Check sheet for the modelled part. Datum: model origin and axes. Units: mm. A direction names the side the tool comes from. Coordinates: 2 decimals unless noted, no trailing zeros. Loops run counter-clockwise (first coordinate to the right, second up) from the corner with the lowest first, then second, coordinate; pieces in that order, holes last. Notation, with made-up numbers: (81.25, 13) - (104.25, 13) arc R24 cw to (104.25, 43) - close; hole circle Ø8 at (-1.75, 1.5). An arc over 180 degrees is marked (long way). Use a Markdown table: item, result. Add a question column.
1) Sectioned sample at C-C, the plane y = 0.65. State how many separate pieces and enclosed holes the cut face has, then the cut area to 3 significant figures.
2) Tool access check on faces 5 (the cylindrical face through (171.507, 1.014, -95.283)), 6 (the flat face through (110, 0, -21)). Record the directions out of +Z, -Z, +X, -X, +Y, -Y that give a thin tool (end or side, any length) a straight path to the whole face; none if there is none.
3) Sectioned sample at A-A, the plane x = 58. Enter the section's corners in (y, z), then the cut area to 3 significant figures.
4) Draft check along X on faces 1 (the cylindrical face through (37.467, 1.014, -69.208)), 2 (the flat face through (201.842, 0.986, 25.333)), 3 (the cylindrical face through (173.347, 1.014, -44.294)), 4 (the flat face through (15.98, 0.99, 25.77)). Enter one of: pulls with the +X half, pulls with the -X half, needs draft (parallel to the pull), parting line crosses it, or undercut.
5) Thickness scan on line 1 (Z direction, x = 96.5, y = 0.3); line 2 (Z direction, x = 72, y = 0.1); line 3 (X direction, y = 1.15, z = -95.5). Record the ranges inside material, lowest first.
6) Go/stop test with flat-tipped pins: P1, Ø2, axis at x = 7.5, z = -9.02, coming from the +Y side; P2, Ø0.6, axis at x = 3.5, y = 1, coming from the -Z side; P3, Ø0.6, axis at y = 1, z = 37, coming from the -X side; P4, Ø1, axis at y = 1, z = -74, coming from the -X side. Record where each tip stops, or that it passes through.
7) Sectioned sample at B-B, the plane x = 17. Enter the section's corners in (y, z), then the cut area to 3 significant figures.
from build123d import *

# Parameters (mm, degrees)
SKETCH_1_R          = 1.7
EXTRUDE_1_DEPTH     = 2
SKETCH_3_R          = 3
CUT_EXTRUDE_1_DEPTH = 10
CUT_EXTRUDE_2_DEPTH = 10


with BuildPart() as part:
    # 草图1 → 凸台-拉伸1 (new body)
    with BuildSketch(Plane(origin=(0, 0, 0), x_dir=(1, 0, 0), z_dir=(0, 1, 0))):
        Polygon((0, -9.790421162), (0, 32.375054838), (13, 32.375054838), (13, 102.375054838), (0, 102.375054838), (0, 144.54053128), (31.526911935, 176.067443214), (73.692388376, 176.067443215), (73.692388376, 163.067443215), (143.692388376, 163.067443215), (143.692388376, 176.067443215), (185.857864376, 176.067443214), (217.384776311, 144.54053128), (217.384776311, 102.375054838), (204.384776311, 102.375054838), (204.384776311, 32.375054838), (217.384776311, 32.375054838), (217.384776311, -9.790421162), (185.857864376, -41.317333096), (143.692388376, -41.317333096), (143.692388376, -26.317333096), (73.692388376, -26.317333096), (73.692388376, -41.317333096), (31.526911935, -41.317333096), align=None)
        with Locations((209.884776311, 9.021225987)):
            Circle(SKETCH_1_R, mode=Mode.SUBTRACT)
        with Locations((209.884776311, 125.728884132)):
            Circle(SKETCH_1_R, mode=Mode.SUBTRACT)
        with Locations((167.046217228, 168.567443215)):
            Circle(SKETCH_1_R, mode=Mode.SUBTRACT)
        with Locations((50.338559083, 168.567443214)):
            Circle(SKETCH_1_R, mode=Mode.SUBTRACT)
        with Locations((7.5, 125.728884132)):
            Circle(SKETCH_1_R, mode=Mode.SUBTRACT)
        with Locations((7.5, 9.021225987)):
            Circle(SKETCH_1_R, mode=Mode.SUBTRACT)
        with Locations((50.338559083, -33.817333096)):
            Circle(SKETCH_1_R, mode=Mode.SUBTRACT)
        with Locations((167.046217228, -33.817333096)):
            Circle(SKETCH_1_R, mode=Mode.SUBTRACT)
    extrude(amount=EXTRUDE_1_DEPTH)

    # 草图3 → 切除-拉伸1 (cut)
    with BuildSketch(Plane(origin=(0, 2, 0), x_dir=(1, 0, 0), z_dir=(0, 1, 0))):
        with Locations((103.610094152, 114.918520178)):
            Circle(SKETCH_3_R)
        with Locations((103.610094152, 24.918520178)):
            Circle(SKETCH_3_R)
        with Locations((193.068894152, 71.918520178)):
            Circle(SKETCH_3_R)
    extrude(amount=-CUT_EXTRUDE_1_DEPTH, mode=Mode.SUBTRACT)

    # 草图4 → 切除-拉伸2 (cut)
    with BuildSketch(Plane(origin=(0, 2, 0), x_dir=(1, 0, 0), z_dir=(0, 1, 0))):
        with BuildLine():
            Line((44.561779376, 103.251399725), (163.361103837, 103.251399725))
            ThreePointArc((163.361103837, 103.251399725), (171.508845116, 95.103658445), (163.361103837, 86.955917166))
            Line((163.361103837, 86.955917166), (44.561779376, 86.955917166))
            ThreePointArc((44.561779376, 86.955917166), (36.414038096, 95.103658445), (44.561779376, 103.251399725))
        make_face()
        with BuildLine():
            Line((45.613100831, 77.534957336), (164.412425292, 77.534957336))
            ThreePointArc((164.412425292, 77.534957336), (172.560166571, 69.387216057), (164.412425292, 61.239474778))
            Line((164.412425292, 61.239474778), (45.613100831, 61.239474778))
            ThreePointArc((45.613100831, 61.239474778), (37.465359552, 69.387216057), (45.613100831, 77.534957336))
        make_face()
        with BuildLine():
            Line((46.401591922, 52.262309138), (165.200916384, 52.262309138))
            ThreePointArc((165.200916384, 52.262309138), (173.348657663, 44.114567858), (165.200916384, 35.966826579))
            Line((165.200916384, 35.966826579), (46.401591922, 35.966826579))
            ThreePointArc((46.401591922, 35.966826579), (38.253850643, 44.114567858), (46.401591922, 52.262309138))
        make_face()
    extrude(amount=-CUT_EXTRUDE_2_DEPTH, mode=Mode.SUBTRACT)


solid = part.part
Solved:
| question | item | result |
|---|---|---|
| 1 | separate pieces | 1 |
| 1 | enclosed holes | 14 |
| 1 | area | 34,900 mm2 |
| 2 | face 5 | +Y, -Y |
| 2 | face 6 | +Z, -Z, +X, -X, -Y |
| 3 | outline | (0, -176.07) - (2, -176.07) - (2, -103.25) - (0, -103.25) - close; (0, -86.96) - (2, -86.96) - (2, -77.53) - (0, -77.53) - close; (0, -61.24) - (2, -61.24) - (2, -52.26) - (0, -52.26) - close; (0, -35.97) - (2, -35.97) - (2, 41.32) - (0, 41.32) - close |
| 3 | area | 337 mm2 |
| 4 | face 1 | undercut |
| 4 | face 2 | pulls with the +X half |
| 4 | face 3 | undercut |
| 4 | face 4 | pulls with the -X half |
| 5 | line 1 | z = -163.07 to -103.25, -86.96 to -77.53, -61.24 to -52.26, -35.97 to 26.32 |
| 5 | line 2 | z = -176.07 to -103.25, -86.96 to -77.53, -61.24 to -52.26, -35.97 to 41.32 |
| 5 | line 3 | x = 13 to 36.42, 171.5 to 204.38 |
| 6 | P1 | passes through |
| 6 | P2 | stops at z = -148.34 |
| 6 | P3 | stops at x = 26.91 |
| 6 | P4 | stops at x = 13 |
| 7 | outline | (0, -161.54) - (2, -161.54) - (2, 26.79) - (0, 26.79) - close |
| 7 | area | 377 mm2 |
